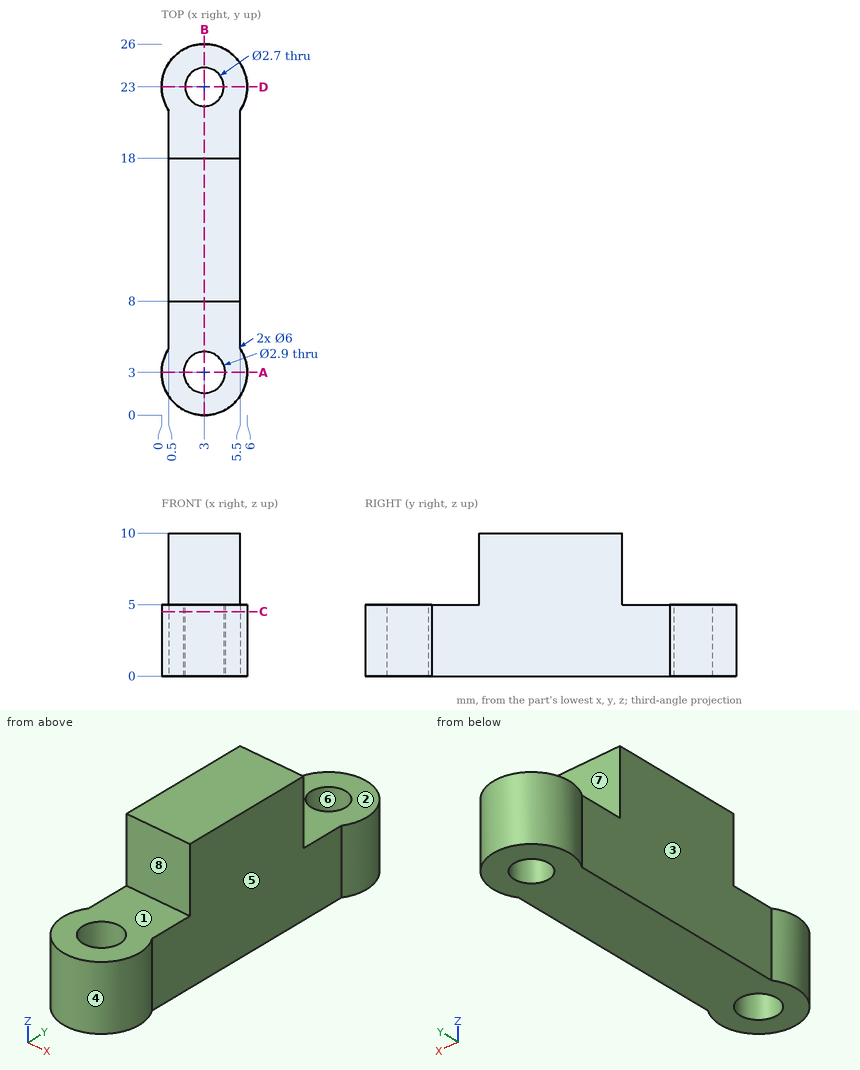
Input: dimensioned drawing with shaded views. Units: mm. Origin: part minimum x, y, z. A direction names the side the tool comes from. Coordinates: 2 decimals unless noted, no trailing zeros. Loops run counter-clockwise (first coordinate to the right, second up) from the corner with the lowest first, then second, coordinate; pieces in that order, holes last.
Q1. Line query: line 1 along Y through (x, z) = (3, 1.35); line 2 along Y through (x, z) = (4, 4); line 3 along Y through (x, z) = (0.8, 7). Output: solid intervals per line, ascending.
Results are:
line 1: y = 0 to 1.55, 4.45 to 21.65, 24.35 to 26
line 2: y = 0.17 to 1.95, 4.05 to 22.09, 23.91 to 25.83
line 3: y = 8 to 18
Q2. Contact query for flat-ended pins moving along their axis: pin 1 (2.5 mm diameter, centred on x = 3.5, z = 6.5, fed in from -Y); pin 2 (4 mm diameter, centred on y = 15.5, z = 3, fed in from -X); pin 3 (1.5 mm diameter, centred on x = 3.5, z = 7.5, fed in from +Y). Output: stop coordinate, or through.
Results are:
pin 1: stops at y = 8
pin 2: stops at x = 0.5
pin 3: stops at y = 18
Q3. Section B-B, the plane x = 3. Return the cut outline in (y, z), and give its area (3 significant figures).
Results are:
outline: (0, 0) - (1.55, 0) - (1.55, 5) - (0, 5) - close; (4.45, 0) - (21.65, 0) - (21.65, 5) - (18, 5) - (18, 10) - (8, 10) - (8, 5) - (4.45, 5) - close; (24.35, 0) - (26, 0) - (26, 5) - (24.35, 5) - close
area: 152 mm2
Q4. Section C-C, the plane z = 4.5. Return the cut outline in (x, y).
Results are:
outline: (0.5, 4.66) arc R3 ccw (long way) to (5.5, 4.66) - (5.5, 21.34) arc R3 ccw (long way) to (0.5, 21.34) - close; hole circle Ø2.9 at (3, 3); hole circle Ø2.7 at (3, 23)
Q5. Section A-A, the plane y = 3. Return the cut outline in (x, z).
Results are:
outline: (0, 0) - (1.55, 0) - (1.55, 5) - (0, 5) - close; (4.45, 0) - (6, 0) - (6, 5) - (4.45, 5) - close
Q6. Mould query, pull axis Y, two halves, no side actions, for the marked faces 6, 7 and 8. Classes: +Y half, -Y half, draft (parallel to the pull), parting line (faces both ways), or undercut.
Results are:
face 6: undercut
face 7: +Y half
face 8: -Y half
Q7. Set-up query: the marked faces 1, 2, 3, 4 and 5. Return all of +Z, -Z, +X, -X, +Y, -Y with unobstructed straight access to the full face (end or side cutting, diameter ignored); none if empty.
Results are:
face 1: +Z, +X, -X, -Y
face 2: +Z, +X, -X, +Y
face 3: +Z, -Z, -X
face 4: +Z, -Z
face 5: +Z, -Z, +X
Q8. Section D-D, the plane y = 23. Return the cut outline in (x, z), and give its area (3 significant figures).
Results are:
outline: (0, 0) - (1.65, 0) - (1.65, 5) - (0, 5) - close; (4.35, 0) - (6, 0) - (6, 5) - (4.35, 5) - close
area: 16.5 mm2
